CAD build for the part. Positions are in the model's coordinates, mm. A direction names the side the tool comes from. Coordinates: 2 decimals unless noted, no trailing zeros. Loops run counter-clockwise (first coordinate to the right, second up) from the corner with the lowest first, then second, coordinate; pieces in that order, holes last. Notation, with made-up numbers: (60.5, 87.5) - (100.5, 87.5) arc R19 cw to (100.5, 106.5) - close; hole circle Ø9 at (36, -8). An arc over 180 degrees is marked (long way). Put each result on its own line as item: value.
```python
from build123d import *

# Parameters (mm, degrees)
SKETCH1_R           = 19.05
BOSS_EXTRUDE1_DEPTH = 46.001643057
FILLET1_R           = 12.7
FILLET2_R           = 2.54


with BuildPart() as part:
    # Sketch1 → Boss-Extrude1 (new body)
    with BuildSketch(Plane.XY):
        with BuildLine():
            Line((101.6, 12.7), (50.8, 12.7))
            Line((50.8, 12.7), (50.8, -12.7))
            Line((50.8, -12.7), (101.6, -12.7))
            Line((101.6, -12.7), (101.6, -38.1))
            Line((101.6, -38.1), (-50.8, -38.1))
            ThreePointArc((-50.8, -38.1), (-88.9, 0), (-50.8, 38.1))
            Line((-50.8, 38.1), (101.6, 38.1))
            Line((101.6, 38.1), (101.6, 12.7))
        make_face()
        with Locations((-50.8, 0)):
            Circle(SKETCH1_R, mode=Mode.SUBTRACT)
    extrude(amount=BOSS_EXTRUDE1_DEPTH)

    # Fillet1
    fillet1_edges = [part.edges().sort_by_distance(p)[0] for p in [
        (101.6, 38.1, 23.000821528),
        (101.6, -38.1, 23.000821528),
    ]]
    fillet(fillet1_edges, radius=FILLET1_R)

    # Fillet2
    fillet2_edges = [part.edges().sort_by_distance(p)[0] for p in [
        (19.05, -38.1, 0),
        (-88.9, 0, 0),
        (76.2, -12.7, 46.001643057),
        (50.8, 12.7, 23.000821528),
        (50.8, -12.7, 23.000821528),
        (50.8, 0, 46.001643057),
        (76.2, 12.7, 46.001643057),
        (101.6, 19.05, 46.001643057),
        (101.6, -19.05, 0),
        (101.6, -19.05, 46.001643057),
        (19.05, 38.1, 0),
        (97.880256121, 34.380256121, 0),
        (97.880256121, -34.380256121, 0),
        (19.05, 38.1, 46.001643057),
        (97.880256121, 34.380256121, 46.001643057),
        (97.880256121, -34.380256121, 46.001643057),
        (-88.9, 0, 46.001643057),
        (19.05, -38.1, 46.001643057),
        (101.6, 19.05, 0),
        (76.2, 12.7, 0),
        (50.8, 0, 0),
        (76.2, -12.7, 0),
    ]]
    fillet(fillet2_edges, radius=FILLET2_R)


solid = part.part
```
Q1. Tool access for faces 4 (the flat face through (77, -12.7, 23)), 5 (the flat face through (18, 38.1, 23)): list every direction of +Z, -Z, +X, -X, +Y, -Y with a clear straight run to the whole face (end or side of a thin tool).
Determined:
face 4: +Z, -Z, +X
face 5: +Z, -Z, +X, -X, +Y
Q2. Mould opens along Y. For faces 1 (the cylindrical face through (-88.89, -0.84, 22.71)), 2 (the cylindrical face through (-33.203, -7.296, 22.679)), 3 (the flat face through (101.6, 19, 23)) say: +Y half, -Y half, draft (parallel to the pull), parting line (faces both ways), or undercut.
Determined:
face 1: parting line
face 2: undercut
face 3: draft
Q3. Wall check: L1, parallel to Y at x = 75, z = 3.5; L2, parallel to X at y = -33, z = 8; L3, parallel to Y at x = 52, z = 20. Give the ranges that are in metal, low to high. Write a range as from..to.
Determined:
L1: -38.1..-12.7, 12.7..38.1
L2: -69.84..99.07
L3: -38.1..-12.32, 12.32..38.1
Q4. Slice it at A-A, the plane z = 4.5. Give the cut face in (x, y), then the cut area to 3 significant figures.
Determined:
outline: (-50.8, -38.1) - (88.9, -38.1) arc R12.7 ccw to (101.6, -25.4) - (101.6, -12.7) - (53.34, -12.7) arc R2.54 cw to (50.8, -10.16) - (50.8, 10.16) arc R2.54 cw to (53.34, 12.7) - (101.6, 12.7) - (101.6, 25.4) arc R12.7 ccw to (88.9, 38.1) - (-50.8, 38.1) arc R38.1 ccw to start; hole circle Ø38.1 at (-50.8, 0)
area: 11,400 mm2
Q5. Slice it at B-B, the plane y = 0. Give the cut face in (x, z).
Determined:
outline: (-88.9, 2.54) arc R2.54 ccw to (-86.36, 0) - (-69.85, 0) - (-69.85, 46) - (-86.36, 46) arc R2.54 ccw to (-88.9, 43.46) - close; (-31.75, 0) - (48.26, 0) arc R2.54 ccw to (50.8, 2.54) - (50.8, 43.46) arc R2.54 ccw to (48.26, 46) - (-31.75, 46) - close
Q6. Pin check, flat tips, straight feed: pin 1 Ø6 at (y, z) = (-4, 28) entering from +X; pin 2 Ø1.5 at (y, z) = (19, 31) entering from -X; pin 3 Ø4 at (y, z) = (4, 41) entering from -X. Stop position of each tip, or through.
Determined:
pin 1: x = 50.8
pin 2: x = -84.24
pin 3: x = -88.85
